Could you check a few things on this model? Use its own coordinates, in mm. Coordinates: 2 decimals unless noted, no trailing zeros. Write each loop counter-clockwise with the first axis right and the second up, starting at its lowest first coordinate (ties: lowest second). Pieces come first, ordered by that corner, then holes. Notation, with made-up numbers: (34, -21) - (39, -21) arc R17 ccw to (39, 5) - close; hole circle Ø8 at (-6, 45.5). An arc over 180 degrees is marked (long way). Answer as a JSON object with one key per item and string values. Group by question number.
1) Please list where these lines run through material, in increasing order: line 1 along X through (y, z) = (0.25, 0.6); line 2 along Y through (x, z) = (1, 0.8); line 3 along Y through (x, z) = (-0.5, 0).
2) If we section it at B-B (z = -0.7): Write out the boundary of the cut face in (x, y).
3) If we section it at C-C (y = 4): Write out the boundary of the cut face in (x, z).
4) Will these pins go through, and if not, where does the flat tip stop? pin 1 Ø1.5 at (y, z) = (5.5, 0.5) entering from +X; pin 2 Ø0.8 at (y, z) = (6, 0) entering from -X; pin 3 Ø0.8 at (y, z) = (-0.5, 0) entering from +X.
5) If we section it at A-A (x = -0.1): Write out the boundary of the cut face in (y, z), plus the area to 3 significant figures.
6) If we section it at D-D (x = 0.6): Write out the boundary of the cut face in (y, z).
```python
from build123d import *
from OCP.BRepFilletAPI import BRepFilletAPI_MakeChamfer

# Parameters (mm, degrees)
SKETCH1_W           = 2.54
SKETCH1_H           = 2.54
BOSS_EXTRUDE1_DEPTH = 2.54
CHAMFER1_SIZE       = 0.4
SKETCH2_W           = 1.74
SKETCH2_H           = 2.54
CUT_EXTRUDE1_DEPTH  = 0.3
SKETCH3_W           = 0.7
SKETCH3_H           = 0.7
BOSS_EXTRUDE2_DEPTH = 5.3
SKETCH4_W           = 0.7
SKETCH4_H           = 0.7
BOSS_EXTRUDE3_DEPTH = 1.55
CHAMFER2_SIZE       = 0.4
CHAMFER2_SIZE2      = 0.122292273


with BuildPart() as part:
    # Sketch1 → Boss-Extrude1 (new body)
    with BuildSketch(Plane(origin=(0, 0, 0), x_dir=(1, 0, 0), z_dir=(0, 1, 0))):
        Rectangle(SKETCH1_W, SKETCH1_H)
    extrude(amount=BOSS_EXTRUDE1_DEPTH)

    # Chamfer1
    chamfer1_edges = [part.edges().sort_by_distance(p)[0] for p in [
        (1.27, 1.27, 1.27),
        (-1.27, 1.27, 1.27),
        (-1.27, 1.27, -1.27),
        (1.27, 1.27, -1.27),
    ]]
    chamfer(chamfer1_edges, length=CHAMFER1_SIZE)

    # Sketch2 → Cut-Extrude1 (cut)
    with BuildSketch(Plane.XZ):
        Rectangle(SKETCH2_W, SKETCH2_H)
    extrude(amount=-CUT_EXTRUDE1_DEPTH, mode=Mode.SUBTRACT)

    # Sketch3 → Boss-Extrude2 (add)
    with BuildSketch(Plane(origin=(0, 2.54, 0), x_dir=(1, 0, 0), z_dir=(0, 1, 0))):
        Rectangle(SKETCH3_W, SKETCH3_H)
    extrude(amount=BOSS_EXTRUDE2_DEPTH)

    # Sketch4 → Boss-Extrude3 (add)
    with BuildSketch(Plane.XZ.offset(-0.3)):
        Rectangle(SKETCH4_W, SKETCH4_H)
    extrude(amount=BOSS_EXTRUDE3_DEPTH)

    # Chamfer2: one chamfer whose edges measure the first distance from different faces: ONE call of the kernel's chamfer builder (chamfer() names one face for all edges)
    chamfer2_edges_1 = [part.edges().sort_by_distance(p)[0] for p in [
        (-0.35, 7.84, 0),
    ]]
    chamfer2_side_1 = [part.faces().sort_by_distance(p)[0] for p in [
        (-0.35, 5.19, 0),
    ]]
    chamfer2_edges_2 = [part.edges().sort_by_distance(p)[0] for p in [
        (0, 7.84, 0.35),
    ]]
    chamfer2_side_2 = [part.faces().sort_by_distance(p)[0] for p in [
        (0, 5.19, 0.35),
    ]]
    chamfer2_edges_3 = [part.edges().sort_by_distance(p)[0] for p in [
        (0.35, 7.84, 0),
    ]]
    chamfer2_side_3 = [part.faces().sort_by_distance(p)[0] for p in [
        (0.35, 5.19, 0),
    ]]
    chamfer2_edges_4 = [part.edges().sort_by_distance(p)[0] for p in [
        (0, 7.84, -0.35),
    ]]
    chamfer2_side_4 = [part.faces().sort_by_distance(p)[0] for p in [
        (0, 5.19, -0.35),
    ]]
    chamfer2_edges_5 = [part.edges().sort_by_distance(p)[0] for p in [
        (0.35, -1.25, 0),
    ]]
    chamfer2_side_5 = [part.faces().sort_by_distance(p)[0] for p in [
        (0.35, -0.475, 0),
    ]]
    chamfer2_edges_6 = [part.edges().sort_by_distance(p)[0] for p in [
        (0, -1.25, 0.35),
    ]]
    chamfer2_side_6 = [part.faces().sort_by_distance(p)[0] for p in [
        (0, -0.475, 0.35),
    ]]
    chamfer2_edges_7 = [part.edges().sort_by_distance(p)[0] for p in [
        (-0.35, -1.25, 0),
    ]]
    chamfer2_side_7 = [part.faces().sort_by_distance(p)[0] for p in [
        (-0.35, -0.475, 0),
    ]]
    chamfer2_edges_8 = [part.edges().sort_by_distance(p)[0] for p in [
        (0, -1.25, -0.35),
    ]]
    chamfer2_side_8 = [part.faces().sort_by_distance(p)[0] for p in [
        (0, -0.475, -0.35),
    ]]
    chamfer2 = BRepFilletAPI_MakeChamfer(part.part.solid().wrapped)
    for e in chamfer2_edges_1:
        chamfer2.Add(CHAMFER2_SIZE, CHAMFER2_SIZE2, e.wrapped, chamfer2_side_1[0].wrapped)  # the first distance lies on this face
    for e in chamfer2_edges_2:
        chamfer2.Add(CHAMFER2_SIZE, CHAMFER2_SIZE2, e.wrapped, chamfer2_side_2[0].wrapped)  # the first distance lies on this face
    for e in chamfer2_edges_3:
        chamfer2.Add(CHAMFER2_SIZE, CHAMFER2_SIZE2, e.wrapped, chamfer2_side_3[0].wrapped)  # the first distance lies on this face
    for e in chamfer2_edges_4:
        chamfer2.Add(CHAMFER2_SIZE, CHAMFER2_SIZE2, e.wrapped, chamfer2_side_4[0].wrapped)  # the first distance lies on this face
    for e in chamfer2_edges_5:
        chamfer2.Add(CHAMFER2_SIZE, CHAMFER2_SIZE2, e.wrapped, chamfer2_side_5[0].wrapped)  # the first distance lies on this face
    for e in chamfer2_edges_6:
        chamfer2.Add(CHAMFER2_SIZE, CHAMFER2_SIZE2, e.wrapped, chamfer2_side_6[0].wrapped)  # the first distance lies on this face
    for e in chamfer2_edges_7:
        chamfer2.Add(CHAMFER2_SIZE, CHAMFER2_SIZE2, e.wrapped, chamfer2_side_7[0].wrapped)  # the first distance lies on this face
    for e in chamfer2_edges_8:
        chamfer2.Add(CHAMFER2_SIZE, CHAMFER2_SIZE2, e.wrapped, chamfer2_side_8[0].wrapped)  # the first distance lies on this face
    add(Compound.cast(chamfer2.Shape()), mode=Mode.REPLACE)


solid = part.part
```
Here are the results:
{
 "1": {"line 1": "x = -1.27 to -0.87, 0.87 to 1.27", "line 2": "y = 0 to 2.54", "line 3": "y = 0.3 to 2.54"},
 "2": {"outline": "(-1.27, 0) - (-0.87, 0) - (-0.87, 0.3) - (0.87, 0.3) - (0.87, 0) - (1.27, 0) - (1.27, 2.54) - (-1.27, 2.54) - close"},
 "3": {"outline": "(-0.35, -0.35) - (0.35, -0.35) - (0.35, 0.35) - (-0.35, 0.35) - close"},
 "4": {"pin 1": "stops at x = 0.35", "pin 2": "stops at x = -0.35", "pin 3": "stops at x = 0.35"},
 "5": {"outline": "(-1.25, -0.23) - (-0.85, -0.35) - (0.3, -0.35) - (0.3, -1.27) - (2.54, -1.27) - (2.54, -0.35) - (7.44, -0.35) - (7.84, -0.23) - (7.84, 0.23) - (7.44, 0.35) - (2.54, 0.35) - (2.54, 1.27) - (0.3, 1.27) - (0.3, 0.35) - (-0.85, 0.35) - (-1.25, 0.23) - close", "area": "10.4 mm²"},
 "6": {"outline": "(0.3, -1.27) - (2.54, -1.27) - (2.54, 1.27) - (0.3, 1.27) - close"}
}
